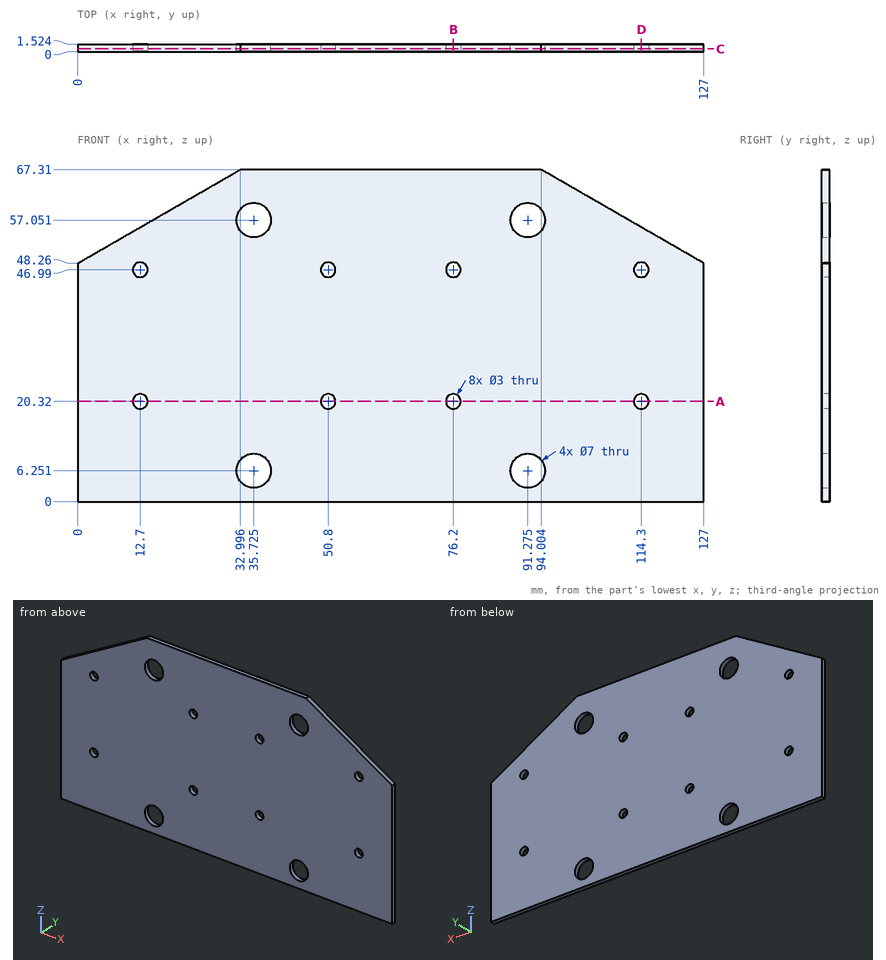
Part print with two shaded views. Sizes in mm from the minimum x, y, z corner. Round coordinates to 2 decimals unless told otherwise and drop trailing zeros. Order: outer loops, then holes, each group sorted by start corner. A loop starts at its lowest first (then second) coordinate and runs counter-clockwise, first axis right, second up.
(1) Band-saw the part on D-D (x = 114.3). List the corners of the cut face in (y, z).
(2) Band-saw the part on B-B (x = 76.2). List the corners of the cut face in (y, z).
(3) Drill centre lines: line 1 (X direction, y = 1, z = 20.32); line 2 (Z direction, x = 76.2, y = 1); line 3 (Z direction, x = 52, y = 1.2). Where is each one in solid material? Low to high.
(4) Pin check, flat tips, straight feed: pin 1 (4 mm diameter, centred on x = 114.3, z = 20.32, fed in from -Y); pin 2 (4 mm diameter, centred on x = 35.72, z = 6.25, fed in from +Y). Stop position of each tip, or through.
(5) Band-saw the part on A-A (z = 20.32). List the corners of the cut face in (x, y), then the cut area to 3 significant figures.
(6) Band-saw the part on C-C (y = 0.55). Give the number of separate pieces and of enclosed holes in the cut face, then the cut area to 3 significant figures.
Verdict:
1. outline: (0, 0) - (1.52, 0) - (1.52, 18.82) - (0, 18.82) - close; (0, 21.82) - (1.52, 21.82) - (1.52, 45.49) - (0, 45.49) - close; (0, 48.49) - (1.52, 48.49) - (1.52, 55.59) - (0, 55.59) - close
2. outline: (0, 0) - (1.52, 0) - (1.52, 18.82) - (0, 18.82) - close; (0, 21.82) - (1.52, 21.82) - (1.52, 45.49) - (0, 45.49) - close; (0, 48.49) - (1.52, 48.49) - (1.52, 67.31) - (0, 67.31) - close
3. line 1: x = 0 to 11.2, 14.2 to 49.3, 52.3 to 74.7, 77.7 to 112.8, 115.8 to 127
3. line 2: z = 0 to 18.82, 21.82 to 45.49, 48.49 to 67.31
3. line 3: z = 0 to 19.42, 21.22 to 46.09, 47.89 to 67.31
4. pin 1: stops at y = 0
4. pin 2: passes through
5. outline: (0, 0) - (11.2, 0) - (11.2, 1.52) - (0, 1.52) - close; (14.2, 0) - (49.3, 0) - (49.3, 1.52) - (14.2, 1.52) - close; (52.3, 0) - (74.7, 0) - (74.7, 1.52) - (52.3, 1.52) - close; (77.7, 0) - (112.8, 0) - (112.8, 1.52) - (77.7, 1.52) - close; (115.8, 0) - (127, 0) - (127, 1.52) - (115.8, 1.52) - close
5. area: 175 mm2
6. separate pieces: 1
6. enclosed holes: 12
6. area: 7,710 mm2
